Source: CAD feature listing. Evaluate the final solid. Frame: model axes, mm. A direction names the side the tool comes from. Give positions to 0.01 mm unless a question says otherwise; leave off trailing zeros. Loops run counter-clockwise (first coordinate to the right, second up) from the corner with the lowest first, then second, coordinate; pieces in that order, holes last.
from build123d import *

# Parameters (mm, degrees)
F1_DEPTH = 13
F2_R     = 31
F3_DEPTH = 8
F4_D     = 50
F6_D     = 11


with BuildPart() as f1:
    # F0 (on Top) → F1 (new body)
    with BuildSketch(Plane.XY):
        with BuildLine():
            Line((37.016888, 44), (-37.016888, 44))
            ThreePointArc((-37.016888, 44), (-39.579121, 41.710228), (-42, 39.271491))
            Line((-42, 39.271491), (-42, -39.271491))
            ThreePointArc((-42, -39.271491), (-39.579121, -41.710228), (-37.016888, -44))
            Line((-37.016888, -44), (37.016888, -44))
            ThreePointArc((37.016888, -44), (39.579121, -41.710228), (42, -39.271491))
            Line((42, -39.271491), (42, 39.271491))
            ThreePointArc((42, 39.271491), (39.579121, 41.710228), (37.016888, 44))
        make_face()
    extrude(amount=F1_DEPTH)

    # F2 (on face) → F3 (join)
    with BuildSketch(Plane.XY.offset(13)):
        Circle(F2_R)
    extrude(amount=F3_DEPTH)

    # F4 (through all)
    with Locations(Plane(origin=(0, 0, 0), x_dir=(1, 0, 0), z_dir=(0, 0, -1))):
        with Locations((0, 0)):
            Hole(F4_D / 2)

    # F6 (through all)
    with Locations(Plane.XY.offset(13)):
        with Locations((-30, 30), (30, 30), (-30, -30), (30, -30)):
            Hole(F6_D / 2)


solid = f1.part
1) Ray query, probe 1 along Y at (x, z) = (-30, 3.5); probe 2 along Y at (x, z) = (0, 6.5); probe 3 along X at (y, z) = (-27.5, 5.5). Return the intervals inside material, ascending.
Checks:
probe 1: y = -44 to -35.5, -24.5 to 24.5, 35.5 to 44
probe 2: y = -44 to -25, 25 to 44
probe 3: x = -42 to -34.9, -25.1 to 25.1, 34.9 to 42
2) Contact query for a flat-ended pin moving along its axis: P1, Ø12.5, axis at x = -30, y = 30, coming from the +Z side. Output: stop coordinate, or through.
Checks:
P1: stops at z = 13
3) Cut plane C-C (z = 3.5). Return loops of the section in (x, y), and give its area (3 significant figures).
Checks:
outline: (-42, -39.27) arc R57.5 ccw to (-37.02, -44) - (37.02, -44) arc R57.5 ccw to (42, -39.27) - (42, 39.27) arc R57.5 ccw to (37.02, 44) - (-37.02, 44) arc R57.5 ccw to (-42, 39.27) - close; hole circle Ø11 at (-30, -30); hole circle Ø11 at (-30, 30); hole circle Ø50 at (0, 0); hole circle Ø11 at (30, -30); hole circle Ø11 at (30, 30)
area: 5,000 mm2
4) Reachability of faces 4 (the cylindrical face through (-4.036, 30.736, 16.944)), 5 (the cylindrical face through (-39.544, 41.743, 6.409)) from +Z, -Z, +X, -X, +Y, -Y: full face, straight path, thin tool, end or side. Return the list, or none.
Checks:
face 4: +Z
face 5: +Z, -Z, -X, +Y
5) Cut plane B-B (x = -30). Return loops of the section in (y, z), and give its area (3 significant figures).
Checks:
outline: (-44, 0) - (-35.5, 0) - (-35.5, 13) - (-44, 13) - close; (-24.5, 0) - (24.5, 0) - (24.5, 13) - (7.81, 13) - (7.81, 21) - (-7.81, 21) - (-7.81, 13) - (-24.5, 13) - close; (35.5, 0) - (44, 0) - (44, 13) - (35.5, 13) - close
area: 983 mm2
6) Cut plane D-D (y = -30). Return loops of the section in (x, z).
Checks:
outline: (-42, 0) - (-35.5, 0) - (-35.5, 13) - (-42, 13) - close; (-24.5, 0) - (24.5, 0) - (24.5, 13) - (7.81, 13) - (7.81, 21) - (-7.81, 21) - (-7.81, 13) - (-24.5, 13) - close; (35.5, 0) - (42, 0) - (42, 13) - (35.5, 13) - close
7) Cut plane A-A (y = 0). Return loops of the section in (x, z).
Checks:
outline: (-42, 0) - (-25, 0) - (-25, 21) - (-31, 21) - (-31, 13) - (-42, 13) - close; (25, 0) - (42, 0) - (42, 13) - (31, 13) - (31, 21) - (25, 21) - close
8) Pull-direction query (Y, two-part tool) for faces 1 (the flat face through (-1, -44, 6)), 2 (the flat face through (-42, 1, 6)), 3 (the cylindrical face through (-23.846, -7.509, 10.647)); classes: released by +Y, released by -Y, zero draft, split by the parting line, or undercut.
Checks:
face 1: released by -Y
face 2: zero draft
face 3: undercut
